Verification items for the finished model (mm, model axes). A direction names the side the tool comes from. Give positions to 0.01 mm unless a question says otherwise; leave off trailing zeros. Write each loop counter-clockwise with the first axis right and the second up, starting at its lowest first coordinate (ties: lowest second). Pieces come first, ordered by that corner, then holes. Notation, with made-up numbers: (0.25, 75.5) -> (49.25, 75.5) arc R19 ccw to (49.25, 105.5) -> close; hole circle Ø8 at (-22, 74). An arc over 180 degrees is marked (long way). Write item = value, one per line.
from build123d import *

# Parameters (mm, degrees)
F1_DEPTH = 52.578
F2_DEPTH = 25.4
F4_DEPTH = 25.4


with BuildPart() as f1:
    # F0 (on Top) → F1 (new body)
    with BuildSketch(Plane.XY):
        with BuildLine():
            ThreePointArc((54.722488, -11.844719), (22.859211, 37.874565), (-35.624544, 29.693728))
            Line((-35.624544, 29.693728), (-14.65048, 29.693728))
            Line((-14.65048, 29.693728), (-14.65048, 27.965855))
            ThreePointArc((-14.65048, 27.965855), (24.269676, 22.947539), (42.420731, -11.844719))
            ThreePointArc((42.420731, -11.844719), (24.269676, -46.636977), (-14.65048, -51.655293))
            Line((-14.65048, -51.655293), (-14.65048, -57.608001))
            Line((-14.65048, -57.608001), (-30.004545, -57.608001))
            ThreePointArc((-30.004545, -57.608001), (26.006031, -59.992793), (54.722488, -11.844719))
        make_face()
        with BuildLine():
            Line((-14.65048, 29.693728), (-35.624544, 29.693728))
            ThreePointArc((-35.624544, 29.693728), (-54.609453, -15.360171), (-30.004545, -57.608001))
            Line((-30.004545, -57.608001), (-14.65048, -57.608001))
            Line((-14.65048, -57.608001), (-14.65048, -51.655293))
            ThreePointArc((-14.65048, -51.655293), (-42.420731, -11.844719), (-14.65048, 27.965855))
            Line((-14.65048, 27.965855), (-14.65048, 29.693728))
        make_face()
    extrude(amount=F1_DEPTH)

    # F0 (on Top) → F2 (join)
    with BuildSketch(Plane.XY):
        with BuildLine():
            Line((-35.624544, 29.693728), (-116.681829, 29.693728))
            Line((-116.681829, 29.693728), (-116.681829, -57.608001))
            Line((-116.681829, -57.608001), (-30.004545, -57.608001))
            ThreePointArc((-30.004545, -57.608001), (-54.609453, -15.360171), (-35.624544, 29.693728))
        make_face()
        with BuildLine():
            ThreePointArc((54.722488, -11.844719), (22.859211, 37.874565), (-35.624544, 29.693728))
            Line((-35.624544, 29.693728), (-14.65048, 29.693728))
            Line((-14.65048, 29.693728), (-14.65048, 27.965855))
            ThreePointArc((-14.65048, 27.965855), (24.269676, 22.947539), (42.420731, -11.844719))
            ThreePointArc((42.420731, -11.844719), (24.269676, -46.636977), (-14.65048, -51.655293))
            Line((-14.65048, -51.655293), (-14.65048, -57.608001))
            Line((-14.65048, -57.608001), (-30.004545, -57.608001))
            ThreePointArc((-30.004545, -57.608001), (26.006031, -59.992793), (54.722488, -11.844719))
        make_face()
    extrude(amount=F2_DEPTH)

    # F3 (on Front) → F4 (join)
    with BuildSketch(Plane.XZ):
        Polygon((-54.646369, 25.746364), (-54.646369, 43.295454), (-84.895462, 25.746364), align=None)
    extrude(amount=F4_DEPTH)


solid = f1.part
Item 1: Sectioned sample at D-D on x = -22.5. Record the cut outline in (y, z), then the cut area to 3 significant figures.
Response values:
outline = (-61.73, 0) -> (-47.81, 0) -> (-47.81, 52.58) -> (-61.73, 52.58) -> close; (24.12, 0) -> (38.04, 0) -> (38.04, 52.58) -> (24.12, 52.58) -> close
area = 1,460 mm^2
Item 2: Sectioned sample at A-A on z = 20. Record the cut outline in (x, y), then the cut area to 3 significant figures.
Response values:
outline = (-116.68, -57.61) -> (-30, -57.61) arc R54.72 ccw (long way) to (-35.62, 29.69) -> (-116.68, 29.69) -> close; hole (-14.65, -51.66) arc R42.42 ccw (long way) to (-14.65, 27.97) arc R42.42 ccw to start
area = 9,740 mm^2
Item 3: Sectioned sample at C-C on y = -36. Record the cut outline in (x, z), then the cut area to 3 significant figures.
Response values:
outline = (-116.68, 0) -> (-34.87, 0) -> (-34.87, 52.58) -> (-49.1, 52.58) -> (-49.1, 25.4) -> (-116.68, 25.4) -> close; (34.87, 0) -> (49.1, 0) -> (49.1, 52.58) -> (34.87, 52.58) -> close
area = 3,210 mm^2
Item 4: Sectioned sample at B-B on x = 0. Record the cut outline in (y, z), then the cut area to 3 significant figures.
Response values:
outline = (-66.57, 0) -> (-54.27, 0) -> (-54.27, 52.58) -> (-66.57, 52.58) -> close; (30.58, 0) -> (42.88, 0) -> (42.88, 52.58) -> (30.58, 52.58) -> close
area = 1,290 mm^2
Item 5: Set-up check for faces 1 (the flat face through (-70, -13, 25.746)), 2 (the flat face through (-63, -25.4, 31)), 3 (the flat face through (-74, -57.608, 13)), 4 (the flat face through (-76, 29.694, 13)): record each of +Z, -Z, +X, -X, +Y, -Y from which the full face is reachable in a straight line by a thin tool's end or side.
Response values:
face_1 = -X, +Y, -Y
face_2 = +Z, -X, -Y
face_3 = +Z, -Z, -X, -Y
face_4 = +Z, -Z, -X, +Y
Item 6: Material ranges on line 1 (X direction, y = -2, z = 26); line 2 (Y direction, x = 1, z = 36); line 3 (Y direction, x = -86, z = 14), recorded low to high.
Response values:
line_1 = -84.46 to -54.65, -53.83 to -41.26, 41.26 to 53.83
line_2 = -66.56 to -54.25, 30.56 to 42.87
line_3 = -57.61 to 29.69
Item 7: Mould release check, pull along X, two halves, no side actions. Record for faces 5 (the flat face through (-69.559, -12.522, 34.644)), 6 (the flat face through (-63, 0, 31)), 7 (the flat face through (-54.646, -4, 34)): +X half, -X half, draft (parallel to the pull), parting line (faces both ways), or undercut.
Response values:
face_5 = -X half
face_6 = draft
face_7 = undercut
Item 8: Go/stop test with flat-tipped pins: P1, Ø4.5, axis at y = -6, z = 31, coming from the +X side; P2, Ø5.5, axis at x = -72.5, z = 32.5, coming from the +Y side; P3, Ø12, axis at y = 25.5, z = 9.5, coming from the +X side. Record where each tip stops, or that it passes through.
Response values:
P1 = 54.6
P2 = 0
P3 = 44.86
